from build123d import *

# Parameters (mm, degrees)
BOSS_EXTRUDE1_DEPTH      = 30
BOSS_EXTRUDE1_DEPTH_BACK = 30


with BuildPart() as part:
    # Sketch1 → Boss-Extrude1 (new body, two sides)
    with BuildSketch(Plane.XY) as boss_extrude1_sk:
        Polygon((-12, -15), (-12, 15), (8, 15), (8, 22.5), (53, 22.5), (53, 27.5), (163, 27.5), (163, 35), (187, 35), (187, 27.5), (297, 27.5), (297, 22.5), (338.5, 22.5), (338.5, 15), (374, 15), (374, -15), (338.5, -15), (338.5, -22.5), (297, -22.5), (297, -27.5), (187, -27.5), (187, -35), (163, -35), (163, -27.5), (53, -27.5), (53, -22.5), (8, -22.5), (8, -15), align=None)
    extrude(amount=BOSS_EXTRUDE1_DEPTH)
    extrude(boss_extrude1_sk.sketch, amount=-BOSS_EXTRUDE1_DEPTH_BACK)

    # Sketch3 → Cut-Revolve2 (revolve, cut)
    with BuildSketch(Plane.XY):
        with BuildLine():
            Line((108.000005708, 22.495261034), (108.000005708, 23.617924612))
            add(Edge.make_bspline(
                [(108.000005708, 23.617924612), (108.69532236, 23.632492565), (110.134086752, 23.662696241), (114.002675386, 23.744055355), (117.52452678, 23.818734211), (122.62413086, 23.927066751), (127.386175822, 24.028960617), (133.517001276, 24.160489916), (140.669558615, 24.314757893), (149.244027294, 24.50035769), (158.933260023, 24.710843629), (169.003951816, 24.929828541), (178.945846596, 25.146047878), (189.059333627, 25.365529494), (198.913066308, 25.578918803), (209.188065069, 25.800360703), (218.243647, 25.994865885), (227.18153574, 26.185528835), (233.191375828, 26.313403618), (238.874035778, 26.433622484), (240.957024273, 26.477631494), (241.999996023, 26.499636974)],
                knots=[0.083332146, 0.083332146, 0.083332146, 0.083332146, 0.083332146, 0.104087624, 0.126568088, 0.157701305, 0.188834523, 0.21996774, 0.251100957, 0.30685696, 0.369123394, 0.431389829, 0.493656263, 0.555922697, 0.618189132, 0.680455566, 0.742722, 0.804988435, 0.85440094, 0.885534157, 0.916667375, 0.916667375, 0.916667375, 0.916667375, 0.916667375], degree=4))
            Line((241.999996023, 26.499636974), (241.999996023, 25.386328483))
            add(Edge.make_bspline(
                [(241.999996023, 25.386328483), (242.997689398, 25.308156454), (244.990789981, 25.150456292), (248.314178963, 24.884174364), (251.097793918, 24.652630256), (254.096338207, 24.40199426), (256.115950151, 24.228401113), (258.395425806, 24.031542714), (260.523519631, 23.843523656), (263.272962125, 23.597575487), (267.617740398, 23.199581767), (272.530644228, 22.731603556), (277.969218388, 22.186806055), (284.502123723, 21.495795918), (289.937964032, 20.886548872), (295.372437907, 20.237558818), (301.88455361, 19.401221609), (308.389001931, 18.498768615), (315.959550127, 17.326428718), (324.308730313, 15.802761995), (331.522595168, 14.182607232), (337.270373253, 12.534677442), (341.314142899, 11.019210316), (343.839526129, 9.821610423), (345.557398761, 8.80275637), (346.740922219, 7.936545395), (347.594801698, 7.171388914), (348.227306411, 6.479610121), (348.723002975, 5.813945223), (349.119004405, 5.147021841), (349.440992029, 4.441727447), (349.699673959, 3.650874012), (349.887237793, 2.736043875), (349.971487339, 1.848234223), (349.997159077, 1.02099573), (350.000343601, 0.437547408), (350.000420527, 0.145847197), (350, 0)],
                knots=[0.085539691, 0.085539691, 0.085539691, 0.085539691, 0.085539691, 0.120111184, 0.154682677, 0.171968424, 0.189254171, 0.206539917, 0.223825664, 0.241111411, 0.258397158, 0.292968652, 0.362111638, 0.396683132, 0.431254625, 0.500397611, 0.534969105, 0.5695406, 0.638683586, 0.707826572, 0.776969547, 0.837594824, 0.8721664, 0.896549847, 0.913250965, 0.925776395, 0.935170687, 0.942808737, 0.949414163, 0.955338894, 0.96134561, 0.967265833, 0.973858415, 0.981569814, 0.990784907, 0.995392454, 1, 1, 1, 1, 1], degree=4))
            Line((350, 0), (0, 0))
            add(Edge.make_bspline(
                [(0, 0), (-0.00035577, 0.120277327), (-0.00031082, 0.360836588), (0.002299922, 0.841992826), (0.022856294, 1.520243321), (0.089579031, 2.24292924), (0.236719839, 2.986493577), (0.43616989, 3.622237895), (0.687299533, 4.198977779), (1.002920086, 4.75468844), (1.407889824, 5.319720548), (1.939569813, 5.917175139), (2.658583589, 6.573081931), (3.67793434, 7.327261742), (5.178835477, 8.218030187), (7.500122996, 9.307468959), (11.351007882, 10.703965668), (16.999713662, 12.236154029), (24.236498755, 13.742442968), (32.666050698, 15.149254822), (41.486862914, 16.386268296), (49.223740463, 17.330086994), (55.862579827, 18.066429658), (61.400762894, 18.639952996), (65.830769492, 19.077356076), (70.267988209, 19.496098455), (74.697234615, 19.8971343), (79.144191725, 20.283849996), (83.564092337, 20.654572527), (87.478187448, 20.970893), (90.760753774, 21.229595839), (93.610940803, 21.448494052), (95.697915689, 21.607520734), (98.724377463, 21.832083001), (101.588044864, 22.043264026), (104.94931787, 22.282042977), (106.985221031, 22.424804888), (108.000005708, 22.495261034)],
                knots=[0, 0, 0, 0, 0, 0.003837631, 0.007675261, 0.015350522, 0.021646811, 0.026957895, 0.031813386, 0.036568429, 0.041680559, 0.047310658, 0.053953193, 0.062039099, 0.07267917, 0.087698911, 0.109550262, 0.143736552, 0.203218265, 0.274262491, 0.345306722, 0.416350952, 0.487395185, 0.522917301, 0.558439418, 0.593961534, 0.629483651, 0.665005767, 0.700527884, 0.73605, 0.771572117, 0.789333175, 0.807094233, 0.824855291, 0.842616349, 0.878138465, 0.913660582, 0.913660582, 0.913660582, 0.913660582, 0.913660582], degree=4))
        make_face()
    revolve(axis=Axis((-1000, 0, 0), (1, 0, 0)), mode=Mode.SUBTRACT)


solid = part.part
Work out the finished part from the listing and answer in its coordinate system (mm). A direction names the side the tool comes from. Give positions to 0.01 mm unless a question says otherwise; leave off trailing zeros. Use a Markdown table: item, result. Add a question column.
1) For a pull along X with two mould halves and no side action, classify faces 1 (the flat face through (338.5, -19, 0)), 2 (the flat face through (241, 27.5, 0)), 3 (the flat face through (108, -21, -9)) as +X half, -X half, draft (parallel to the pull), parting line (faces both ways), or undercut.
2) Consider line 1 along Z through (x, y) = (202.5, -2.5); line 2 along X through (y, z) = (-5.5, 3.5); line 3 along Z through (x, y) = (163, 16). Determine where each line is inside the solid, lowest interval first.
3) Which of the six approach directions +Z, -Z, +X, -X, +Y, -Y give full straight-line access (tool end or side, diameter ignored) to faces 4 (the flat face through (317, 22.5, 0)), 5 (the flat face through (31, -22.5, 0)), 6 (the flat face through (243, -27.5, 0))?
4) Each of these flat-tipped pins is pushed along its axis until it touches: P1, Ø2, axis at y = 30.5, z = -10.5, coming from the +X side; P2, Ø8, axis at x = 296, z = -19, coming from the -Y side; P3, Ø4, axis at y = -25.5, z = -5.5, coming from the +X side. Where does it stop, or does it pass through?
Reported:
| question | item | result |
|---|---|---|
| 1 | face 1 | +X half |
| 1 | face 2 | draft |
| 1 | face 3 | undercut |
| 2 | line 1 | z = -30 to -25.53, 25.53 to 30 |
| 2 | line 2 | x = -12 to 2.63, 348.17 to 374 |
| 2 | line 3 | z = -30 to -18.95, 18.95 to 30 |
| 3 | face 4 | +Z, -Z, +X, +Y |
| 3 | face 5 | +Z, -Z, -X, -Y |
| 3 | face 6 | +Z, -Z, +X, -Y |
| 4 | P1 | stops at x = 187 |
| 4 | P2 | stops at y = -27.5 |
| 4 | P3 | stops at x = 297 |
